from build123d import *

# Parameters (mm, degrees)
SKETCH_1_R                     = 3
SKETCH_1_W                     = 73
SKETCH_1_H                     = 23.2
EXTRUDE_1_DEPTH                = 2
FILLET_1_R                     = 1
HOLE_WIZARD_M2_5_1_D           = 2.7
HOLE_WIZARD_M2_5_1_DEPTH       = 5.538838164
HOLE_WIZARD_M2_5_1_CSINK_D     = 5.5
HOLE_WIZARD_M2_5_1_CSINK_ANGLE = 90
HOLE_WIZARD_M2_5_1_TIP         = 0.811161836
CHAMFER_1_SIZE                 = 0.2


with BuildPart() as part:
    # 草图1 → 凸台-拉伸1 (new body)
    with BuildSketch(Plane.XY):
        with Locations((-26.4, 11.6)):
            Circle(SKETCH_1_R)
        with Locations((-12, 11.6)):
            Circle(SKETCH_1_R)
        with Locations((12, 11.6)):
            Circle(SKETCH_1_R)
        with Locations((26.4, 11.6)):
            Circle(SKETCH_1_R)
        with Locations((26.4, -11.6)):
            Circle(SKETCH_1_R)
        with Locations((12, -11.6)):
            Circle(SKETCH_1_R)
        with Locations((-12, -11.6)):
            Circle(SKETCH_1_R)
        with Locations((-26.4, -11.6)):
            Circle(SKETCH_1_R)
        Rectangle(SKETCH_1_W, SKETCH_1_H)
    extrude(amount=EXTRUDE_1_DEPTH)

    # 圆角1
    fillet_1_edges = [part.edges().sort_by_distance(p)[0] for p in [
        (29.4, 11.6, 1),
        (23.4, 11.6, 1),
        (23.4, -11.6, 1),
        (29.4, -11.6, 1),
        (9, -11.6, 1),
        (15, -11.6, 1),
        (-15, -11.6, 1),
        (-9, -11.6, 1),
        (-29.4, -11.6, 1),
        (-23.4, -11.6, 1),
        (-23.4, 11.6, 1),
        (-29.4, 11.6, 1),
        (-9, 11.6, 1),
        (-15, 11.6, 1),
        (-36.5, -11.6, 1),
        (36.5, -11.6, 1),
        (36.5, 11.6, 1),
        (-36.5, 11.6, 1),
        (9, 11.6, 1),
        (15, 11.6, 1),
    ]]
    fillet(fillet_1_edges, radius=FILLET_1_R)

    # M2.5 锥坑平头螺钉的锥形沉头孔1
    with Locations(Plane(origin=(-26.4, 11.6, 2), x_dir=(1, 0, 0), z_dir=(0, 0, 1))):
        with Locations((0, 0), (14.4, 0), (38.4, 0), (52.8, 0), (52.8, -23.2), (38.4, -23.2), (14.4, -23.2), (0, -23.2)):
            CounterSinkHole(HOLE_WIZARD_M2_5_1_D / 2, HOLE_WIZARD_M2_5_1_CSINK_D / 2, depth=HOLE_WIZARD_M2_5_1_DEPTH, counter_sink_angle=HOLE_WIZARD_M2_5_1_CSINK_ANGLE)
            with Locations((0, 0, -(HOLE_WIZARD_M2_5_1_DEPTH + HOLE_WIZARD_M2_5_1_TIP / 2))):  # 118° drill point
                Cone(0, HOLE_WIZARD_M2_5_1_D / 2, HOLE_WIZARD_M2_5_1_TIP, mode=Mode.SUBTRACT)

    # 倒角1
    chamfer_1_edges = [part.edges().sort_by_distance(p)[0] for p in [
        (-36.5, 0, 2),
        (-32.886491673, -11.6, 2),
        (-26.4, -14.6, 2),
        (-19.2, -11.6, 2),
        (-12, -14.6, 2),
        (0, -11.6, 2),
        (12, -14.6, 2),
        (19.2, -11.6, 2),
        (26.4, -14.6, 2),
        (32.886491673, -11.6, 2),
        (36.207106781, -11.307106781, 2),
        (-36.207106781, 11.307106781, 2),
        (-36.207106781, -11.307106781, 2),
        (36.207106781, 11.307106781, 2),
        (15.260610911, 11.809430585, 0),
        (15.260610911, 11.809430585, 2),
        (23.139389089, 11.809430585, 0),
        (23.139389089, 11.809430585, 2),
        (29.660610911, 11.809430585, 0),
        (29.660610911, 11.809430585, 2),
        (29.660610911, -11.809430585, 0),
        (29.660610911, -11.809430585, 2),
        (23.139389089, -11.809430585, 0),
        (23.139389089, -11.809430585, 2),
        (15.260610911, -11.809430585, 0),
        (15.260610911, -11.809430585, 2),
        (8.739389089, -11.809430585, 0),
        (8.739389089, -11.809430585, 2),
        (-8.739389089, -11.809430585, 0),
        (-8.739389089, -11.809430585, 2),
        (-15.260610911, -11.809430585, 0),
        (-15.260610911, -11.809430585, 2),
        (-23.139389089, -11.809430585, 0),
        (-23.139389089, -11.809430585, 2),
        (-29.660610911, -11.809430585, 0),
        (-29.660610911, -11.809430585, 2),
        (-29.660610911, 11.809430585, 0),
        (-29.660610911, 11.809430585, 2),
        (-23.139389089, 11.809430585, 2),
        (-23.139389089, 11.809430585, 0),
        (-15.260610911, 11.809430585, 0),
        (-15.260610911, 11.809430585, 2),
        (-8.739389089, 11.809430585, 2),
        (-8.739389089, 11.809430585, 0),
        (8.739389089, 11.809430585, 0),
        (8.739389089, 11.809430585, 2),
        (12, 14.6, 0),
        (12, 14.6, 2),
        (19.2, 11.6, 2),
        (19.2, 11.6, 0),
        (26.4, 14.6, 0),
        (26.4, 14.6, 2),
        (32.886491673, 11.6, 2),
        (32.886491673, 11.6, 0),
        (36.5, 0, 0),
        (32.886491673, -11.6, 0),
        (26.4, -14.6, 0),
        (19.2, -11.6, 0),
        (12, -14.6, 0),
        (0, -11.6, 0),
        (-12, -14.6, 0),
        (-19.2, -11.6, 0),
        (-26.4, -14.6, 0),
        (-32.886491673, -11.6, 0),
        (-36.5, 0, 0),
        (-32.886491673, 11.6, 0),
        (-26.4, 14.6, 0),
        (-19.2, 11.6, 0),
        (-12, 14.6, 0),
        (0, 11.6, 0),
        (36.207106781, -11.307106781, 0),
        (-36.207106781, 11.307106781, 0),
        (-36.207106781, -11.307106781, 0),
        (36.207106781, 11.307106781, 0),
        (36.5, 0, 2),
        (0, 11.6, 2),
        (-12, 14.6, 2),
        (-19.2, 11.6, 2),
        (-26.4, 14.6, 2),
        (-32.886491673, 11.6, 2),
    ]]
    chamfer(chamfer_1_edges, length=CHAMFER_1_SIZE)


solid = part.part
Could you check a few things on this model? Use its own coordinates, in mm. A direction names the side the tool comes from. Round coordinates to 2 decimals unless told otherwise and drop trailing zeros. Order: outer loops, then holes, each group sorted by start corner. A loop starts at its lowest first (then second) coordinate and runs counter-clockwise, first axis right, second up. Notation, with made-up numbers: M -19,-22.75 L 7,-22.75 A24 ccw 7,15.25 Z; hole C 23.25,84 d4. An arc over 180 degrees is marked long. One line per item, written item: value.
(1) Imagine slicing it at A-A (x = -26.4). Write out the boundary of the cut face in (y, z).
Ans:
outline: M -14.6,0.2 L -14.4,0 L -12.95,0 L -12.95,0.6 L -14.35,2 L -14.4,2 L -14.6,1.8 Z; M -10.25,0 L 10.25,0 L 10.25,0.6 L 8.85,2 L -8.85,2 L -10.25,0.6 Z; M 12.95,0 L 14.4,0 L 14.6,0.2 L 14.6,1.8 L 14.4,2 L 14.35,2 L 12.95,0.6 Z
(2) I'm going to push flat-ended pins straight in: P1, Ø1, axis at x = 25, z = 0.5, coming from the +Y side; P2, Ø0.5, axis at x = 19, z = 1.5, coming from the +Y side; P3, Ø1.6, axis at x = 12, y = 11.6, coming from the +Z side; P4, Ø0.8, axis at x = -2.5, z = 1, coming from the -Y side. Where does each tip first touch, or does it pass through?
Ans:
P1: stops at y = 14.46
P2: stops at y = 11.6
P3: passes through
P4: stops at y = -11.6
(3) Imagine slicing it at B-B (x = 21.5). Write out the boundary of the cut face in (y, z), and give its area (3 significant figures).
Ans:
outline: M -11.6,0.2 L -11.4,0 L 11.4,0 L 11.6,0.2 L 11.6,1.8 L 11.4,2 L -11.4,2 L -11.6,1.8 Z
area: 46.3 mm^2
(4) Which directions (+Z, -Z, +X, -X, +Y, -Y) give clear straight access to the entire face, cutting with the end or side of a thin tool? Please do faces 1 (the flat face through (0, -11.6, 1)), 2 (the flat face through (-33, -11.6, 1)), 3 (the flat face through (-33, 11.6, 1)).
Ans:
face 1: +Z, -Z, -Y
face 2: +Z, -Z, -X, -Y
face 3: +Z, -Z, -X, +Y
(5) If we mould it in two halves opening along X, with no side actions, what happens to faces 4 (the cylindrical face through (-27.647, -12.117, 0.296)), 5 (the flat face through (-1, 0, 2))? For each: released by +X, released by -X, zero draft, split by the parting line, or undercut.
Ans:
face 4: undercut
face 5: zero draft
(6) Imagine slicing it at C-C (z = 1.25). Count the separate pieces of the cut face and the enclosed holes in it, and give its area (3 significant figures).
Ans:
separate pieces: 1
enclosed holes: 8
area: 1,710 mm^2
(7) I need wall thicknesses on line 1 along Y through (x, z) = (-26.4, 0.3); line 2 along Y through (x, z) = (-11, 0.8); line 3 along Y through (x, z) = (33.5, 1.35). Which ranges of each line are inside material? Lowest first, please. Write a range as from..to.
Ans:
line 1: y = -14.6..-12.95, -10.25..10.25, 12.95..14.6
line 2: y = -14.43..-12.78, -10.42..10.42, 12.78..14.43
line 3: y = -11.6..11.6
